from build123d import *

# Parameters (mm, degrees)
F1_DEPTH = 1149.7084
F3_D     = 11


with BuildPart() as f1:
    # F0 (on Right) → F1 (new body)
    with BuildSketch(Plane.YZ):
        with BuildLine():
            ThreePointArc((11.35, 18.857143), (10.764214, 20.271356), (9.35, 20.857143))
            Line((9.35, 20.857143), (-9.65, 20.857143))
            ThreePointArc((-9.65, 20.857143), (-11.064214, 20.271356), (-11.65, 18.857143))
            Line((-11.65, 18.857143), (-11.65, -17.142857))
            ThreePointArc((-11.65, -17.142857), (-11.064214, -18.557071), (-9.65, -19.142857))
            Line((-9.65, -19.142857), (9.35, -19.142857))
            ThreePointArc((9.35, -19.142857), (10.764214, -18.557071), (11.35, -17.142857))
            Line((11.35, -17.142857), (11.35, -9.142857))
            Line((11.35, -9.142857), (9.85, -9.142857))
            Line((9.85, -9.142857), (9.85, -16.642857))
            ThreePointArc((9.85, -16.642857), (9.557107, -17.349964), (8.85, -17.642857))
            Line((8.85, -17.642857), (-9.15, -17.642857))
            ThreePointArc((-9.15, -17.642857), (-9.857107, -17.349964), (-10.15, -16.642857))
            Line((-10.15, -16.642857), (-10.15, 18.357143))
            ThreePointArc((-10.15, 18.357143), (-9.857107, 19.06425), (-9.15, 19.357143))
            Line((-9.15, 19.357143), (8.85, 19.357143))
            ThreePointArc((8.85, 19.357143), (9.557107, 19.06425), (9.85, 18.357143))
            Line((9.85, 18.357143), (9.85, 10.857143))
            Line((9.85, 10.857143), (11.35, 10.857143))
            Line((11.35, 10.857143), (11.35, 18.857143))
        make_face()
    extrude(amount=F1_DEPTH)

    # F3 (through all)
    with Locations(Plane.XZ.offset(11.65)):
        with Locations((20, 0.857143), (1129.7084, 0.857143)):
            Hole(F3_D / 2)


solid = f1.part
Build history of the part. All positions in model axes, mm. A direction names the side the tool comes from. Give positions to 0.01 mm unless a question says otherwise; leave off trailing zeros. Order: outer loops, then holes, each group sorted by start corner. A loop starts at its lowest first (then second) coordinate and runs counter-clockwise, first axis right, second up. Notation, with made-up numbers: M -22.5,-6.5 L -1.5,-6.5 A16 cw -1.5,11.5 Z; hole C 26.25,18.25 d5. An arc over 180 degrees is marked long. Put each result on its own line as item: value.
Item 1: Two-plate mould, pull along Z, no slides. Class faces 3 (the flat face through (567, 0, 20.857)), 4 (the flat face through (567, -10.15, 1)), 5 (the flat face through (1149.708, -10.4, -0.5)): +Z half, -Z half, draft (parallel to the pull), parting line (faces both ways), or undercut.
From the geometry:
face 3: +Z half
face 4: undercut
face 5: draft
Item 2: Slice it at B-B, the plane x = 631.5. Write the cut outline in (y, z).
From the geometry:
outline: M -11.65,-17.14 A2 ccw -9.65,-19.14 L 9.35,-19.14 A2 ccw 11.35,-17.14 L 11.35,-9.14 L 9.85,-9.14 L 9.85,-16.64 A1 cw 8.85,-17.64 L -9.15,-17.64 A1 cw -10.15,-16.64 L -10.15,18.36 A1 cw -9.15,19.36 L 8.85,19.36 A1 cw 9.85,18.36 L 9.85,10.86 L 11.35,10.86 L 11.35,18.86 A2 ccw 9.35,20.86 L -9.65,20.86 A2 ccw -11.65,18.86 Z
Item 3: 3-axis set-ups, long thin cutter, end or side, ignore diameter. For faces 1 (the flat face through (0, -10.4, -0.5)), 2 (the flat face through (567, 0, 19.357)): which of +Z, -Z, +X, -X, +Y, -Y reach the whole face in a straight line?
From the geometry:
face 1: +Z, -Z, -X, +Y, -Y
face 2: +X, -X
Item 4: Flat gauge pins, fed straight in: pin 1 Ø1.6 at (x, y) = (528, 11) entering from +Z; pin 2 Ø1.2 at (x, y) = (749, 10.5) entering from -Z. Where does each tip first touch, or does it go through?
From the geometry:
pin 1: stops at z = 20.67
pin 2: stops at z = -19.07
Item 5: Slice it at A-A, the plane y = -5.25. Write the cut outline in (x, z), plus the area to 3 significant figures.
From the geometry:
outline: M 0,-19.14 L 1149.71,-19.14 L 1149.71,-17.64 L 0,-17.64 Z; M 0,19.36 L 1149.71,19.36 L 1149.71,20.86 L 0,20.86 Z
area: 3,450 mm2
Item 6: Probe line 1 (Z direction, x = 1011, y = -4.75); line 2 (Y direction, x = 983.5, z = 12.5); line 3 (Z direction, x = 833.5, y = 10). List the from-to ranges inside material, lowest first. Write a range as [from, to].
From the geometry:
line 1: z = [-19.14, -17.64], [19.36, 20.86]
line 2: y = [-11.65, -10.15], [9.85, 11.35]
line 3: z = [-19.03, -9.14], [10.86, 20.75]
